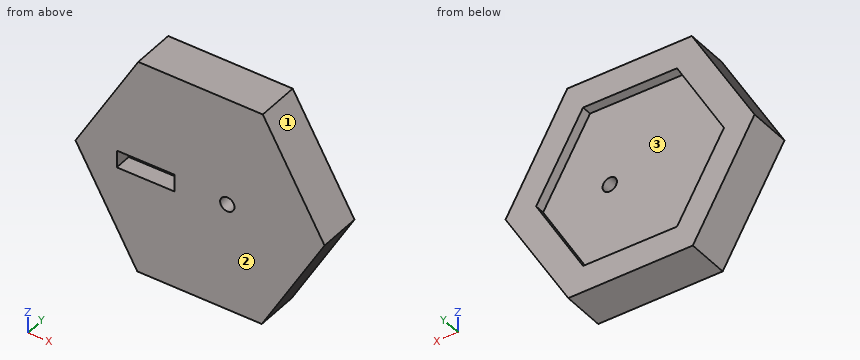
```python
from build123d import *

# Parameters (mm, degrees)
F1_DEPTH = 7.62
F2_R     = 1.27
F3_DEPTH = 25.4
F4_W     = 10.240057
F4_H     = 3.056733
F5_DEPTH = 3.048
F7_DEPTH = 1.778


with BuildPart() as f1:
    # F0 (on Front) → F1 (new body)
    with BuildSketch(Plane.XZ):
        Polygon((-22.053678, 0.098198), (-11.111881, -19.049946), (10.941797, -19.148145), (22.053678, -0.098198), (11.111881, 19.049946), (-10.941797, 19.148145), align=None)
    extrude(amount=F1_DEPTH)

    # F2 (on face) → F3 (cut)
    with BuildSketch(Plane.XZ.offset(7.62)):
        with Locations((4.827668, 0)):
            Circle(F2_R)
    extrude(amount=-F3_DEPTH, mode=Mode.SUBTRACT)

    # F4 (on face) → F5 (cut)
    with BuildSketch(Plane.XZ.offset(7.62)):
        with Locations((-9.62871, -0.152837)):
            Rectangle(F4_W, F4_H)
    extrude(amount=-F5_DEPTH, mode=Mode.SUBTRACT)

    # F6 (on Front) → F7 (cut)
    with BuildSketch(Plane.XZ):
        Polygon((-8.3185, -14.408065), (8.3185, -14.408065), (16.637, 0), (8.3185, 14.408065), (-8.3185, 14.408065), (-16.637, 0), align=None)
    extrude(amount=F7_DEPTH, mode=Mode.SUBTRACT)


solid = f1.part
```
The model under review builds one solid part; all positions refer to its coordinate system, in mm. Face numbers are marked on the shaded views. Round coordinates to 2 decimals unless told otherwise and drop trailing zeros. Loops run counter-clockwise (first coordinate to the right, second up) from the corner with the lowest first, then second, coordinate; pieces in that order, holes last. Notation, with made-up numbers: (39, 88.5) -> (78, 88.5) arc R16 cw to (78, 96.5) -> close; hole circle Ø11 at (37.5, -3.75). An arc over 180 degrees is marked (long way). Answer in a Markdown table with one row per item.
1) Draft analysis for pull direction Z (two halves, no side actions). For the marked faces 1, 2 and 3, state which applies: pulls with the +Z half, pulls with the -Z half, needs draft (parallel to the pull), parting line crosses it, or undercut.
Taken from the geometry:
| item | result |
|---|---|
| face 1 | pulls with the +Z half |
| face 2 | needs draft |
| face 3 | undercut |
2) Consider section A-A, the plane y = -2.5. Write out the cut boundary in (x, z).
Taken from the geometry:
| item | result |
|---|---|
| outline | (-22.05, 0.1) -> (-11.11, -19.05) -> (10.94, -19.15) -> (22.05, -0.1) -> (11.11, 19.05) -> (-10.94, 19.15) -> close; hole circle Ø2.54 at (4.83, 0) |
3) Consider section B-B, the plane y = -5.75. Write out the cut boundary in (x, z), plus the area to 3 significant figures.
Taken from the geometry:
| item | result |
|---|---|
| outline | (-22.05, 0.1) -> (-11.11, -19.05) -> (10.94, -19.15) -> (22.05, -0.1) -> (11.11, 19.05) -> (-10.94, 19.15) -> close; hole (-14.75, -1.68) -> (-4.51, -1.68) -> (-4.51, 1.38) -> (-14.75, 1.38) -> close; hole circle Ø2.54 at (4.83, 0) |
| area | 1,230 mm² |
4) Wall thickness on line 1 along Y through (x, z) = (2, 12); line 2 along X through (y, z) = (-5.75, 6); line 3 along Z through (x, y) = (20.5, -2.25): over which ranges is each line inside the solid? List them lowest first.
Taken from the geometry:
| item | result |
|---|---|
| line 1 | y = -7.62 to -1.78 |
| line 2 | x = -18.61 to 18.57 |
| line 3 | z = -2.76 to 2.62 |
5) Consider section D-D, the plane z = 3.5. Write out the cut boundary in (x, y), plus the area to 3 significant figures.
Taken from the geometry:
| item | result |
|---|---|
| outline | (-20.07, -7.62) -> (20, -7.62) -> (20, 0) -> (14.62, 0) -> (14.62, -1.78) -> (-14.62, -1.78) -> (-14.62, 0) -> (-20.07, 0) -> close |
| area | 253 mm² |
6) For pin 1 Ø2 at (y, z) = (-6.5, -2.5) entering from +X; pin 2 Ø4 at (y, z) = (-6.5, -2.5) entering from -X; pin 3 Ø0.9 at (x, z) = (-8, -1) entering from -Y, all flat-tipped, find the tip position at first contact; note any pin that passes through.
Taken from the geometry:
| item | result |
|---|---|
| pin 1 | stops at x = 21.24 |
| pin 2 | stops at x = -21.71 |
| pin 3 | stops at y = -4.57 |
7) Consider section C-C, the plane x = -14. Write out the cut boundary in (y, z), plus the area to 3 significant figures.
Taken from the geometry:
| item | result |
|---|---|
| outline | (-7.62, -14) -> (0, -14) -> (0, -4.57) -> (-1.78, -4.57) -> (-1.78, 4.57) -> (0, 4.57) -> (0, 13.91) -> (-7.62, 13.91) -> (-7.62, 1.38) -> (-4.57, 1.38) -> (-4.57, -1.68) -> (-7.62, -1.68) -> close |
| area | 187 mm² |
